Here's the drawing with two shaded views (mm, measured from the low corner). I have some questions. A direction names the side the tool comes from. Give positions to 0.01 mm unless a question says otherwise; leave off trailing zeros. Loops run counter-clockwise (first coordinate to the right, second up) from the corner with the lowest first, then second, coordinate; pieces in that order, holes last. Notation, with made-up numbers: (60, 53) - (94, 53) arc R24 cw to (94, 76) - close; hole circle Ø4 at (-33, -37.5). An arc over 180 degrees is marked (long way). Write each question's results on one line, items separated by ' | '. Start each with the question number.
1) If I drill on probe 1 along X at (y, z) = (25.4, 5.75); probe 2 along Y at (x, z) = (38.1, 5.25); probe 3 along X at (y, z) = (14, 5.5) (1 decimal), over which ranges is the centre line in solid material (lowest first)? Write a range as [from, to].
2) I want a section at D-D, the plane z = 3. Write out the boundary of the cut face in (x, y), and give its area (3 significant figures).
3) I'm going to push flat-ended pins straight in: pin 1 (2.5 mm diameter, centred on x = 63, z = 11.5, fed in from -Y); pin 2 (4 mm diameter, centred on x = 40, y = 6.5, fed in from +Z). Where does each tip first touch, or does it pass through?
4) I want a section at B-B, the plane z = 11.75. Write out the boundary of the cut face in (x, y).
5) If we mould it in two halves opening along Y, with no side actions, what happens to the marked faces 4, 5 and 6? For each: +Y half, -Y half, draft (parallel to the pull), parting line (faces both ways), or undercut.
6) I want a section at A-A, the plane x = 38.1. Write out the boundary of the cut face in (y, z), and give its area (3 significant figures).
7) I want a section at C-C, the plane y = 25.4. Write out the boundary of the cut face in (x, z).
8) On a 3-axis mill with a long thin cutter (end or side, diameter ignored), from which of +Z, -Z, +X, -X, +Y, -Y can I reach the whole of each face in a straight line? I mean the marked faces 1, 2 and 3. Say none if no direction works.
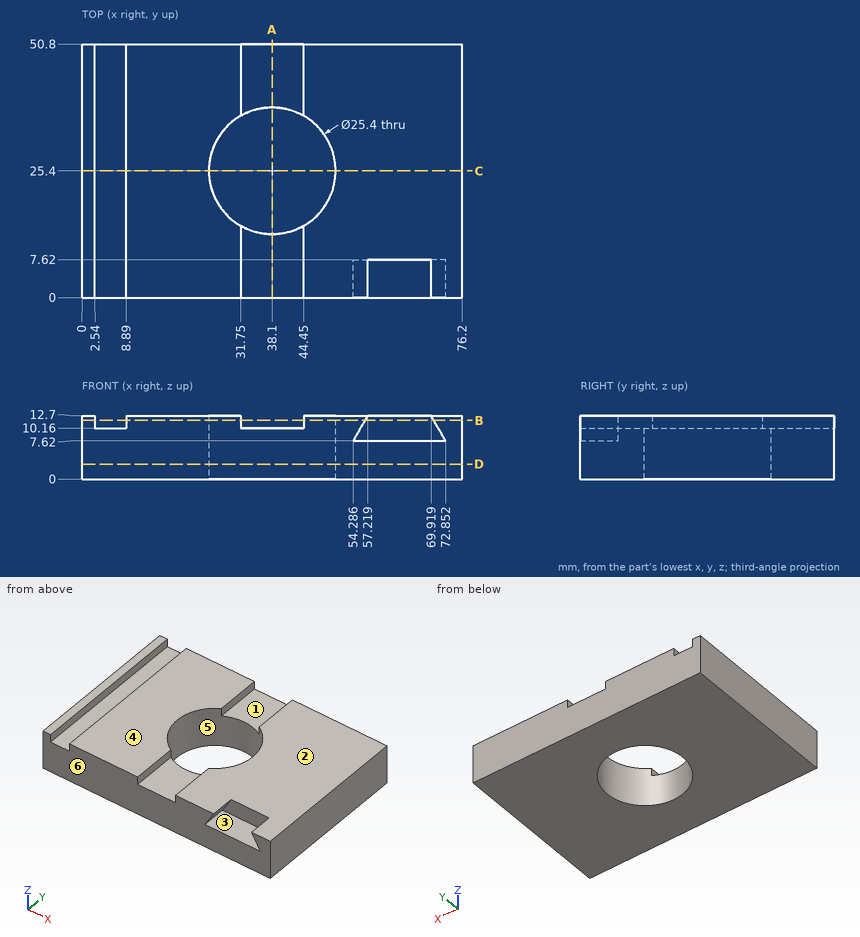
Answers:
1) probe 1: x = [0, 25.4], [50.8, 76.2] | probe 2: y = [0, 12.7], [38.1, 50.8] | probe 3: x = [0, 32.5], [43.7, 76.2]
2) outline: (0, 0) - (76.2, 0) - (76.2, 50.8) - (0, 50.8) - close; hole circle Ø25.4 at (38.1, 25.4) | area: 3,360 mm2
3) pin 1: stops at y = 7.62 | pin 2: stops at z = 10.16
4) outline: (0, 0) - (2.54, 0) - (2.54, 50.8) - (0, 50.8) - close; (8.89, 0) - (31.75, 0) - (31.75, 14.4) arc R12.7 cw to (31.75, 36.4) - (31.75, 50.8) - (8.89, 50.8) - close; (44.45, 0) - (56.67, 0) - (56.67, 7.62) - (70.47, 7.62) - (70.47, 0) - (76.2, 0) - (76.2, 50.8) - (44.45, 50.8) - (44.45, 36.4) arc R12.7 cw to (44.45, 14.4) - close
5) face 4: draft | face 5: undercut | face 6: -Y half
6) outline: (0, 0) - (12.7, 0) - (12.7, 10.16) - (0, 10.16) - close; (38.1, 0) - (50.8, 0) - (50.8, 10.16) - (38.1, 10.16) - close | area: 258 mm2
7) outline: (0, 0) - (25.4, 0) - (25.4, 12.7) - (8.89, 12.7) - (8.89, 10.16) - (2.54, 10.16) - (2.54, 12.7) - (0, 12.7) - close; (50.8, 0) - (76.2, 0) - (76.2, 12.7) - (50.8, 12.7) - close
8) face 1: +Z, +Y, -Y | face 2: +Z, +X, -X, +Y, -Y | face 3: -Y
